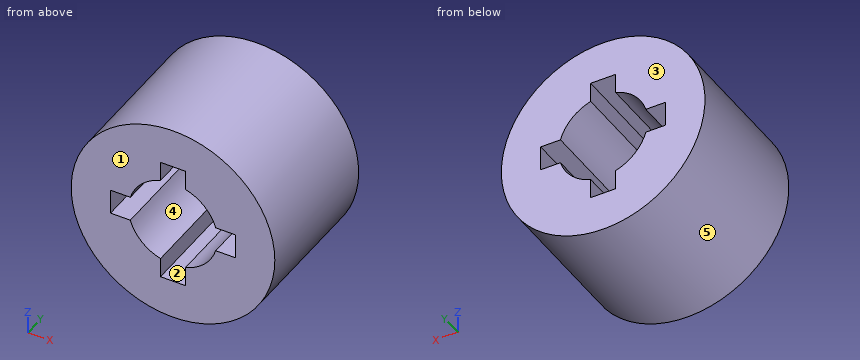
```python
from build123d import *

# Parameters (mm, degrees)
F0_R     = 4.075
F1_DEPTH = 5.75


with BuildPart() as f1:
    # F0 (on Front) → F1 (new body)
    with BuildSketch(Plane.XZ):
        Circle(F0_R)
        with BuildLine():
            Line((-0.5, 2.5), (0.5, 2.5))
            Line((0.5, 2.5), (0.5, 1.708333))
            ThreePointArc((0.5, 1.708333), (1.25865, 1.25865), (1.708333, 0.5))
            Line((1.708333, 0.5), (2.5, 0.5))
            Line((2.5, 0.5), (2.5, -0.5))
            Line((2.5, -0.5), (1.708333, -0.5))
            ThreePointArc((1.708333, -0.5), (1.25865, -1.25865), (0.5, -1.708333))
            Line((0.5, -1.708333), (0.5, -2.5))
            Line((0.5, -2.5), (-0.5, -2.5))
            Line((-0.5, -2.5), (-0.5, -1.708333))
            ThreePointArc((-0.5, -1.708333), (-1.25865, -1.25865), (-1.708333, -0.5))
            Line((-1.708333, -0.5), (-2.5, -0.5))
            Line((-2.5, -0.5), (-2.5, 0.5))
            Line((-2.5, 0.5), (-1.708333, 0.5))
            ThreePointArc((-1.708333, 0.5), (-1.25865, 1.25865), (-0.5, 1.708333))
            Line((-0.5, 1.708333), (-0.5, 2.5))
        make_face(mode=Mode.SUBTRACT)
    extrude(amount=F1_DEPTH)


solid = f1.part
```
Design review of the part built by this model. Coordinates are the model's own, in mm. Face numbers are marked on the shaded views. A direction names the side the tool comes from. Coordinates: 2 decimals unless noted, no trailing zeros. Loops run counter-clockwise (first coordinate to the right, second up) from the corner with the lowest first, then second, coordinate; pieces in that order, holes last. Notation, with made-up numbers: (-21.5, 23.5) -> (-13.5, 23.5) arc R22 ccw to (-13.5, 56.5) -> close; hole circle Ø2 at (-4, 88.25). An arc over 180 degrees is marked (long way). Answer as a JSON object with one key per item and string values.
Q1. Take a section at C-C on z = 0. Give the boundary of the cut face in (x, y) (3 decimals).
Answer block:
{"outline": "(-4.075, -5.75) -> (-2.5, -5.75) -> (-2.5, 0) -> (-4.075, 0) -> close; (2.5, -5.75) -> (4.075, -5.75) -> (4.075, 0) -> (2.5, 0) -> close"}
Q2. Take a section at A-A on x = 0. Give the boundary of the cut face in (y, z) (3 decimals), plus the area to 3 significant figures.
Answer block:
{"outline": "(-5.75, -4.075) -> (0, -4.075) -> (0, -2.5) -> (-5.75, -2.5) -> close; (-5.75, 2.5) -> (0, 2.5) -> (0, 4.075) -> (-5.75, 4.075) -> close", "area": "18.1 mm^2"}
Q3. Take a section at D-D on x = -3.5. Give the boundary of the cut face in (y, z).
Answer block:
{"outline": "(-5.75, -2.09) -> (0, -2.09) -> (0, 2.09) -> (-5.75, 2.09) -> close"}
Q4. Take a section at B-B on y = -0.5. Give the boundary of the cut face in (x, z) (3 decimals).
Answer block:
{"outline": "circle Ø8.15 at (0, 0); hole (-2.5, -0.5) -> (-1.708, -0.5) arc R1.78 ccw to (-0.5, -1.708) -> (-0.5, -2.5) -> (0.5, -2.5) -> (0.5, -1.708) arc R1.78 ccw to (1.708, -0.5) -> (2.5, -0.5) -> (2.5, 0.5) -> (1.708, 0.5) arc R1.78 ccw to (0.5, 1.708) -> (0.5, 2.5) -> (-0.5, 2.5) -> (-0.5, 1.708) arc R1.78 ccw to (-1.708, 0.5) -> (-2.5, 0.5) -> close"}
Q5. Tool access review of the marked faces 1 and 2: name each direction out of +Z, -Z, +X, -X, +Y, -Y from which nothing blocks a thin tool from reaching the whole face with its end or side.
Answer block:
{"face 1": "+Z, -Z, +X, -X, -Y", "face 2": "+Y, -Y"}
Q6. To check wall thickness, follow L1, parallel to X at y = -2.7, z = -2; L2, parallel to Z at x = 1, y = -5.5; L3, parallel to X at y = -1.1, z = 0.25. State the ranges of each line that lie inside material, in increasing order.
Answer block:
{"L1": "x = -3.55 to -0.5, 0.5 to 3.55", "L2": "z = -3.95 to -1.47, 1.47 to 3.95", "L3": "x = -4.07 to -2.5, 2.5 to 4.07"}
Q7. The part is to be moulded in two halves that separate along Z. For the marked faces 3, 4 and 5, say which applies: +Z half, -Z half, draft (parallel to the pull), parting line (faces both ways), or undercut.
Answer block:
{"face 3": "draft", "face 4": "undercut", "face 5": "parting line"}
Q8. Clearance check with flat-ended pins moving along their axes: pin 1 Ø0.9 at (y, z) = (-3, 2) entering from +X; pin 2 Ø0.9 at (y, z) = (-1.5, -2) entering from -X; pin 3 Ø0.9 at (x, y) = (2, -3) entering from -Z; pin 4 Ø1 at (x, z) = (0, -0.5) entering from -Y. State where each tip first meets the part, or that it passes through.
Answer block:
{"pin 1": "stops at x = 3.77", "pin 2": "stops at x = -3.77", "pin 3": "stops at z = -3.77", "pin 4": "passes through"}
